from build123d import *

# Parameters (mm, degrees)
SKETCH_1_W          = 20
SKETCH_1_H          = 10
EXTRUDE_1_DEPTH     = 17
SKETCH_2_R          = 2
CUT_EXTRUDE_1_DEPTH = 29.08914381
M3X0_5_1_D          = 2.5
M3X0_5_1_DEPTH      = 12.5
M3X0_5_1_TIP        = 0.751075774
M3X0_5_2_REACH      = 30.089
M3X0_5_2_BORE_R     = 1.25


with BuildPart() as part:
    # ｽｹｯﾁ1 → ﾎﾞｽ - 押し出し1 (new body)
    with BuildSketch(Plane.XY):
        with Locations((10, 5)):
            Rectangle(SKETCH_1_W, SKETCH_1_H)
    extrude(amount=EXTRUDE_1_DEPTH)

    # ｽｹｯﾁ2 → ｶｯﾄ - 押し出し1 (cut, through all)
    with BuildSketch(Plane.XZ):
        with Locations(Location((10, 10, 0), (0, 0, 270))):
            Circle(SKETCH_2_R)
    extrude(amount=-CUT_EXTRUDE_1_DEPTH, mode=Mode.SUBTRACT)

    # M3x0.5 ねじ穴1
    with Locations(Plane(origin=(0, 0, 0), x_dir=(-1, 0, 0), z_dir=(0, 0, -1))):
        with Locations((-5, 5), (-15, 5)):
            Hole(M3X0_5_1_D / 2, depth=M3X0_5_1_DEPTH)
            with Locations((0, 0, -(M3X0_5_1_DEPTH + M3X0_5_1_TIP / 2))):  # 118° drill point
                Cone(0, M3X0_5_1_D / 2, M3X0_5_1_TIP, mode=Mode.SUBTRACT)

    # M3x0.5 ねじ穴2 bore → M3x0.5 ねじ穴2 (cut, up to next)
    with BuildSketch(Plane.XY.offset(17), mode=Mode.PRIVATE) as m3x0_5_2_sk1:
        with Locations((10, 5)):
            Circle(M3X0_5_2_BORE_R)
    m3x0_5_2_tool1 = extrude(m3x0_5_2_sk1.sketch, amount=-M3X0_5_2_REACH, mode=Mode.PRIVATE) & part.part
    add(m3x0_5_2_tool1.solids().sort_by_distance((10, 5, 17))[0], mode=Mode.SUBTRACT)


solid = part.part
Geometry: final body of the model. Coordinates: model frame, mm. A direction names the side the tool comes from. Coordinates: 2 decimals unless noted, no trailing zeros. Loops run counter-clockwise (first coordinate to the right, second up) from the corner with the lowest first, then second, coordinate; pieces in that order, holes last. Notation, with made-up numbers: M 61.5,71 L 100.5,71 A21 ccw 100.5,97 Z; hole C 64.25,-7 d1. An arc over 180 degrees is marked long. One line per item, written item: value. Start each with the question number.
1) Cut plane A-A (z = 10). Return loops of the section in (x, y), then the cut area to 3 significant figures.
2) Pin query (flat end, axial travel): P1, Ø6, axis at x = 13, z = 2, coming from the -Y side; P2, Ø1.5, axis at x = 10, y = 5, coming from the +Z side; P3, Ø2, axis at x = 15, y = 5, coming from the -Z side; P4, Ø1.5, axis at x = 5, y = 5, coming from the -Z side. Return the tip coordinate at first contact, or that it passes through.
3) Draft query along Y for faces 1 (the conical face through (5.16, 5.15, 13.12)), 2 (the flat face through (0, 5, 8)), 3 (the flat face through (10, 10, 6)). Return one class per face: released by +Y, released by -Y, zero draft, split by the parting line, or undercut.
4) Cut plane C-C (y = 7.5). Return loops of the section in (x, z), then the cut area to 3 significant figures.
5) Cut plane D-D (z = 4.5). Return loops of the section in (x, y).
6) Cut plane B-B (x = 10). Return loops of the section in (y, z).
7) Material intervals for L1, parallel to X at y = 5, z = 3.5; L2, parallel to Y at x = 10, z = 15.55; L3, parallel to X at y = 0.75, z = 10, sorted ascending. Write a range as from..to.
8) Reachability of faces 4 (the flat face through (10, 5, 0)), 5 (the cylindrical face through (9.84, 6.24, 14.32)), 6 (the cylindrical face through (14.73, 3.78, 6.34)) from +Z, -Z, +X, -X, +Y, -Y: full face, straight path, thin tool, end or side. Return the list, or none.
Evaluation:
1. outline: M 0,0 L 8,0 L 8,10 L 0,10 Z; M 12,0 L 20,0 L 20,10 L 12,10 Z; hole C 5,5 d2.5; hole C 15,5 d2.5
1. area: 150 mm^2
2. P1: y = 0
2. P2: z = 8.15
2. P3: z = 12.65
2. P4: z = 12.8
3. face 1: undercut
3. face 2: zero draft
3. face 3: released by +Y
4. outline: M 0,0 L 20,0 L 20,17 L 0,17 Z; hole C 10,10 d4
4. area: 327 mm^2
5. outline: M 0,0 L 20,0 L 20,10 L 0,10 Z; hole C 5,5 d2.5; hole C 15,5 d2.5
6. outline: M 0,0 L 10,0 L 10,8 L 0,8 Z; M 0,12 L 3.75,12 L 3.75,17 L 0,17 Z; M 6.25,12 L 10,12 L 10,17 L 6.25,17 Z
7. L1: 0..3.75, 6.25..13.75, 16.25..20
7. L2: 0..3.75, 6.25..10
7. L3: 0..8, 12..20
8. face 4: -Z, +X, -X, +Y, -Y
8. face 5: +Z
8. face 6: -Z
